Can you work these out from the model? Positions are in its coordinate system, mm. Face numbers are marked on the shaded views. A direction names the side the tool comes from. Round coordinates to 2 decimals unless told otherwise and drop trailing zeros. Loops run counter-clockwise (first coordinate to the right, second up) from the corner with the lowest first, then second, coordinate; pieces in that order, holes last. Notation, with made-up numbers: (87.5, -2.75) -> (125.5, -2.75) arc R20 cw to (125.5, 22.25) -> close; hole circle Ø8 at (59.5, 26.25). An arc over 180 degrees is marked (long way). Answer as a JSON object with one key per item and string values.
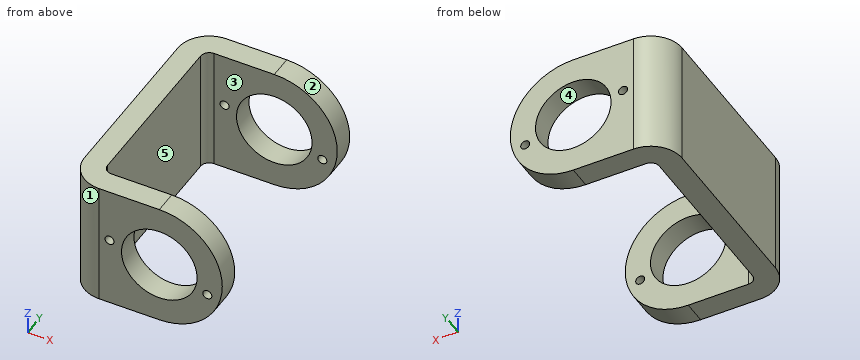
```python
from build123d import *

# Parameters (mm, degrees)
BASE_FLANGE1_DEPTH        = 17.5
FILLET3_RADIUS            = 17.5
FILLET3_LENGTH            = 6.35
FILLET4_RADIUS            = 17.5
FILLET4_LENGTH            = 6.35
CUT_EXTRUDE6_DEPTH        = 57.670097935
CUT_EXTRUDE6_DEPTH_BACK   = 57.670097935
SKETCH23_R                = 10.5
M3X0_5_TAPPED_HOLE1_D     = 2.5
M3X0_5_TAPPED_HOLE1_DEPTH = 6.35
M3X0_5_TAPPED_HOLE2_D     = 2.5


# Sheet-metal steps are written as plain solids
with BuildPart() as part:
    # Sketch20 → Base-Flange1 (new, symmetric)
    with BuildSketch(Plane.XY):
        with BuildLine():
            Line((43, -32.5), (8.730000066, -32.5))
            ThreePointArc((8.730000066, -32.5), (2.55695782, -29.94304218), (0, -23.769999934))
            Line((0, -23.769999934), (0, 23.769999934))
            ThreePointArc((0, 23.769999934), (2.55695782, 29.94304218), (8.730000066, 32.5))
            Line((8.730000066, 32.5), (43, 32.5))
            Line((43, 32.5), (43, 26.15))
            Line((43, 26.15), (8.730000066, 26.15))
            ThreePointArc((8.730000066, 26.15), (7.04708588, 25.45291412), (6.35, 23.769999934))
            Line((6.35, 23.769999934), (6.35, -23.769999934))
            ThreePointArc((6.35, -23.769999934), (7.04708588, -25.45291412), (8.730000066, -26.15))
            Line((8.730000066, -26.15), (43, -26.15))
            Line((43, -26.15), (43, -32.5))
        make_face()
    extrude(amount=BASE_FLANGE1_DEPTH, both=True)

    # Fillet3: full round fillet: the end face becomes a half cylinder, R = half its width
    fillet3_face = Plane((43, 29.325, 0), x_dir=(0, 1, 0), z_dir=(1, 0, 0))  # on the end face: x along it, z out of the body
    fillet3_slab = fillet3_face.offset(-FILLET3_RADIUS / 2) * Box(FILLET3_LENGTH, 2 * FILLET3_RADIUS, FILLET3_RADIUS, mode=Mode.PRIVATE)  # the body's end, R deep
    fillet3_round = Plane((25.5, 29.325, 0), x_dir=(1, 0, 0), z_dir=(0, 1, 0)) * Cylinder(FILLET3_RADIUS, FILLET3_LENGTH, mode=Mode.PRIVATE)  # its axis R under the face
    add(fillet3_slab - fillet3_round, mode=Mode.SUBTRACT)

    # Fillet4: full round fillet: the end face becomes a half cylinder, R = half its width
    fillet4_face = Plane((43, -29.325, 0), x_dir=(0, 1, 0), z_dir=(1, 0, 0))  # on the end face: x along it, z out of the body
    fillet4_slab = fillet4_face.offset(-FILLET4_RADIUS / 2) * Box(FILLET4_LENGTH, 2 * FILLET4_RADIUS, FILLET4_RADIUS, mode=Mode.PRIVATE)  # the body's end, R deep
    fillet4_round = Plane((25.5, -29.325, 0), x_dir=(1, 0, 0), z_dir=(0, 1, 0)) * Cylinder(FILLET4_RADIUS, FILLET4_LENGTH, mode=Mode.PRIVATE)  # its axis R under the face
    add(fillet4_slab - fillet4_round, mode=Mode.SUBTRACT)

    # Sketch23 → Cut-Extrude6 (cut, two sides: drawn at the far end of the back side and taken through both)
    with BuildSketch(Plane(origin=(0, 0, 0), x_dir=(1, 0, 0), z_dir=(0, 1, 0)).offset(-CUT_EXTRUDE6_DEPTH_BACK)):
        with Locations(Location((25.5, 0, 0), (0, 0, 270))):
            Circle(SKETCH23_R)
    extrude(amount=CUT_EXTRUDE6_DEPTH + CUT_EXTRUDE6_DEPTH_BACK, mode=Mode.SUBTRACT)

    # M3x0.5 Tapped Hole1
    with Locations(Plane(origin=(0, 32.5, 0), x_dir=(1, 0, 0), z_dir=(0, 1, 0))):
        with Locations((38.85199985, 4.21), (11.681986395, -2.25)):
            Hole(M3X0_5_TAPPED_HOLE1_D / 2, depth=M3X0_5_TAPPED_HOLE1_DEPTH)

    # M3x0.5 Tapped Hole2 (through all)
    with Locations(Plane(origin=(0, -32.5, 0), x_dir=(-1, 0, 0), z_dir=(0, -1, 0))):
        with Locations((-11.681986395, -2.25), (-38.85199985, 4.21)):
            Hole(M3X0_5_TAPPED_HOLE2_D / 2)


solid = part.part
```
Q1. I'm going to push flat-ended pins straight in: pin 1 (19 mm diameter, centred on x = 25.5, z = 0, fed in from -Y); pin 2 (1.5 mm diameter, centred on y = -1, z = -7.5, fed in from +X). Where does each tip first touch, or does it pass through?
Determined:
{"pin 1": "through", "pin 2": "x = 6.35"}
Q2. If I drill on L1, parallel to Y at x = 31, z = 12.5; L2, parallel to X at y = -28, z = -4.21, over which ranges is the centre line in solid material (lowest first)? Write a range as [from, to].
Determined:
{"L1": "[-32.5, -26.15], [26.15, 32.5]", "L2": "[1.09, 15.88], [35.12, 37.6], [40.1, 42.49]"}
Q3. We'd pull the mould along Y, two halves only. Please class the marked faces 1, 2 and 3: pulls with the +Y half, pulls with the -Y half, needs draft (parallel to the pull), parting line crosses it, or undercut.
Determined:
{"face 1": "pulls with the -Y half", "face 2": "needs draft", "face 3": "undercut"}
Q4. I want a section at C-C, the plane z = -4.21. Write out the boundary of the cut face in (x, y), then the cut area to 3 significant figures.
Determined:
{"outline": "(0, -23.77) arc R8.73 ccw to (8.73, -32.5) -> (15.88, -32.5) -> (15.88, -26.15) -> (8.73, -26.15) arc R2.38 cw to (6.35, -23.77) -> (6.35, 23.77) arc R2.38 cw to (8.73, 26.15) -> (15.88, 26.15) -> (15.88, 32.5) -> (8.73, 32.5) arc R8.73 ccw to (0, 23.77) -> close; (35.12, -32.5) -> (37.6, -32.5) -> (37.6, -26.15) -> (35.12, -26.15) -> close; (35.12, 26.15) -> (37.6, 26.15) -> (37.6, 32.5) -> (35.12, 32.5) -> close; (40.1, -32.5) -> (42.49, -32.5) -> (42.49, -26.15) -> (40.1, -26.15) -> close; (40.1, 26.15) -> (42.49, 26.15) -> (42.49, 32.5) -> (40.1, 32.5) -> close", "area": "565 mm²"}
Q5. I want a section at B-B, the plane x = 23. Write out the boundary of the cut face in (y, z), then the cut area to 3 significant figures.
Determined:
{"outline": "(-32.5, -17.5) -> (-26.15, -17.5) -> (-26.15, -10.2) -> (-32.5, -10.2) -> close; (-32.5, 10.2) -> (-26.15, 10.2) -> (-26.15, 17.5) -> (-32.5, 17.5) -> close; (26.15, -17.5) -> (32.5, -17.5) -> (32.5, -10.2) -> (26.15, -10.2) -> close; (26.15, 10.2) -> (32.5, 10.2) -> (32.5, 17.5) -> (26.15, 17.5) -> close", "area": "185 mm²"}
Q6. I want a section at A-A, the plane z = 0. Write out the boundary of the cut face in (x, y), then the cut area to 3 significant figures.
Determined:
{"outline": "(0, -23.77) arc R8.73 ccw to (8.73, -32.5) -> (15, -32.5) -> (15, -26.15) -> (8.73, -26.15) arc R2.38 cw to (6.35, -23.77) -> (6.35, 23.77) arc R2.38 cw to (8.73, 26.15) -> (15, 26.15) -> (15, 32.5) -> (8.73, 32.5) arc R8.73 ccw to (0, 23.77) -> close; (36, -32.5) -> (43, -32.5) -> (43, -26.15) -> (36, -26.15) -> close; (36, 26.15) -> (43, 26.15) -> (43, 32.5) -> (36, 32.5) -> close", "area": "581 mm²"}
Q7. On a 3-axis mill with a long thin cutter (end or side, diameter ignored), from which of +Z, -Z, +X, -X, +Y, -Y can I reach the whole of each face in a straight line? I mean the marked faces 4 and 5. Say none if no direction works.
Determined:
{"face 4": "+Y, -Y", "face 5": "+Z, -Z, +X"}
Q8. I want a section at D-D, the plane y = -12. Write out the boundary of the cut face in (x, z).
Determined:
{"outline": "(0, -17.5) -> (6.35, -17.5) -> (6.35, 17.5) -> (0, 17.5) -> close"}
